Autodesk Fusion 360 part; units mm, degrees
sketch "Sketch1" plane through (0, 0, 0) normal (1, 0, 0) x (0, 0, -1)
  circle A0 centre (-25, 15) radius 20
  dimension "d1" = 40
extrude "Extrude1" add sketch "Sketch1" along normal blind 5
fillet "Fillet1" radius 2 1 edges at (5, 7.7677, 43.6465)
fillet "Fillet2" radius 2 1 edges at (0, 7.7677, 43.6465)
sketch "Sketch2" plane through (5, 0, 0) normal (1, 0, 0) x (0, 0, -1)
  circle A0 centre (-25, 15) radius 18
  circle A1 centre (-25, 15) radius 5
  dimension "d6" = 10
extrude "Extrude2" add sketch "Sketch2" along normal blind 30 contours A1
thread "Thread1"
sketch "Sketch3" plane through (0, 0, 0) normal (1, 0, 0) x (0, 0, -1)
sketch "Sketch4" plane through (0, 0, 0) normal (-1, 0, 0) x (0, 0, 1)
  circle A0 centre (25, 15) radius 18
sketch "Sketch5" plane through (0, 0, 0) normal (0, 0, 1) x (1, 0, 0)
sketch "Sketch6" plane through (0, 0, 0) normal (0, 0, 1) x (1, 0, 0)
  line L0 (-10, 15) -> (50, 15)
  line L1 (0, 0) -> (0, 29.9666)
  arc A0 (0, 29.9666) -> (0, 0.0334) centre (-10, 15) ccw
  dimension "d9" = 36
extrude "Extrude3" add sketch "Sketch6" along normal blind 3 from surface at 23.5
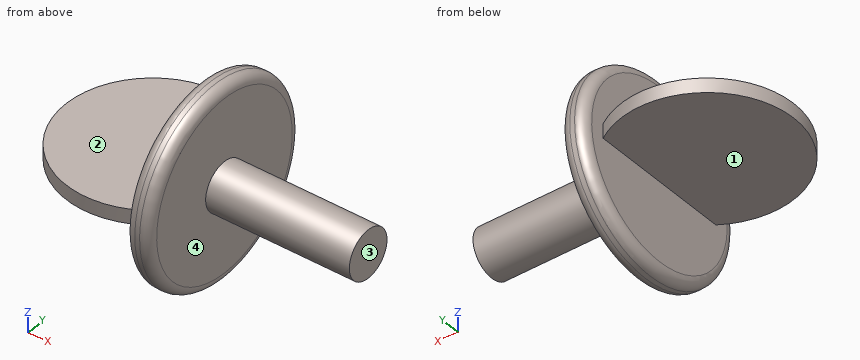
Could you check a few things on this model? Use its own coordinates, in mm. Face numbers are marked on the shaded views. A direction names the side the tool comes from. Round coordinates to 2 decimals unless told otherwise and drop trailing zeros. Loops run counter-clockwise (first coordinate to the right, second up) from the corner with the lowest first, then second, coordinate; pieces in that order, holes last.
Q1. I want a section at A-A (y = 15). Write out the boundary of the cut face in (x, z).
Q2. On a 3-axis mill with a long thin cutter (end or side, diameter ignored), from which of +Z, -Z, +X, -X, +Y, -Y can I reach the whole of each face in a straight line? I mean the marked faces 1, 2, 3 and 4. Say none if no direction works.
Q3. I want a section at D-D (x = -10). Write out the boundary of the cut face in (y, z).
Q4. Please list where these lines run through material, in increasing order: L1, parallel to Z at x = -14.5, y = 17; L2, parallel to X at y = 29.5, z = 28; L3, parallel to Z at x = 31, y = 16.
Q5. I want a section at B-B (z = 25). Write out the boundary of the cut face in (x, y), and give its area (3 significant figures).
Q6. I want a section at C-C (x = 15). Write out the boundary of the cut face in (y, z).
Q7. For P1, Ø5, axis at x = -17.5, y = 19.5, coming from the -Z side; P2, Ø8, axis at x = 2.5, z = 21.5, coming from the -Y side; P3, Ø6, axis at x = -1.5, z = 21, coming from the +Y side; P4, Ø18, axis at y = 20.5, z = 21.5, coming from the -X side, each with a flat end and sliding along its axis, tell me the tip position at first contact or that it passes through.
Answer below:
1. outline: (-28, 23.5) - (0, 23.5) - (0, 7) arc R2 ccw to (2, 5) - (3, 5) arc R2 ccw to (5, 7) - (5, 20) - (35, 20) - (35, 30) - (5, 30) - (5, 43) arc R2 ccw to (3, 45) - (2, 45) arc R2 ccw to (0, 43) - (0, 26.5) - (-28, 26.5) - close
2. face 1: -Z, -X, +Y, -Y
2. face 2: +Z, -X, +Y, -Y
2. face 3: +Z, -Z, +X, +Y, -Y
2. face 4: +X
3. outline: (-3, 23.5) - (33, 23.5) - (33, 26.5) - (-3, 26.5) - close
4. L1: z = 23.5 to 26.5
4. L2: x = 0 to 5
4. L3: z = 20.1 to 29.9
5. outline: (0, -3) arc R2 ccw to (2, -5) - (3, -5) arc R2 ccw to (5, -3) - (5, 10) - (35, 10) - (35, 20) - (5, 20) - (5, 33) arc R2 ccw to (3, 35) - (2, 35) arc R2 ccw to (0, 33) - (0, 29.97) arc R18 ccw (long way) to (0, 0.03) - close
5. area: 1,350 mm2
6. outline: circle Ø10 at (15, 25)
7. P1: stops at z = 23.5
7. P2: stops at y = -5
7. P3: stops at y = 34.66
7. P4: stops at x = -28
